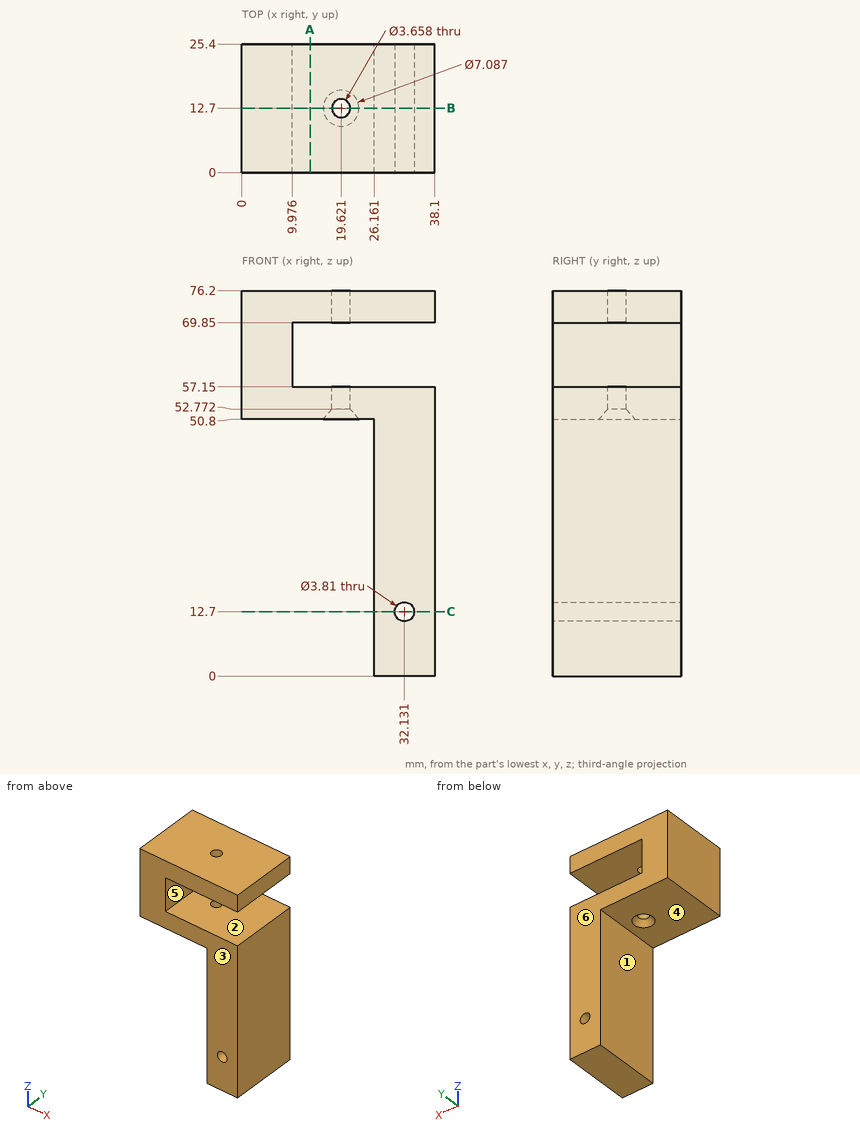
Part print with two shaded views. Sizes in mm from the minimum x, y, z corner. A direction names the side the tool comes from. Give positions to 0.01 mm unless a question says otherwise; leave off trailing zeros. Order: outer loops, then holes, each group sorted by start corner. A loop starts at its lowest first (then second) coordinate and runs counter-clockwise, first axis right, second up.
(1) Tool access for the marked faces 1, 2 and 3: list every direction of +Z, -Z, +X, -X, +Y, -Y with a clear straight run to the whole face (end or side of a thin tool).
(2) Saw through at C-C, the plane z = 12.7. Give the cut face in (x, y) (1 decimal).
(3) Saw through at A-A, the plane x = 13.5. Give the cut face in (y, z).
(4) Drill centre lines: L1, parallel to Z at x = 28, y = 15.25; L2, parallel to Z at x = 21.5, y = 16; L3, parallel to X at y = 6, z = 12.7 (1 decimal). Where is each one in solid material? Low to high.
(5) Flat gauge pins, fed straight in: pin 1 (10 mm diameter, centred on y = 13, z = 19, fed in from -X); pin 2 (12.5 mm diameter, centred on x = 11, y = 18.5, fed in from -Z); pin 3 (6.5 mm diameter, centred on y = 8, z = 65.5, fed in from +X). Where does each tip first touch, or does it go through?
(6) Mould opens along Z. For the marked faces 4, 5 and 6 say: released by +Z, released by -Z, zero draft, split by the parting line, or undercut.
(7) Saw through at B-B, the plane y = 12.7. State how many separate pieces and enclosed holes the cut face has, then the cut area to 3 significant figures.
Results found:
1. face 1: -Z, -X, +Y, -Y
1. face 2: +X, +Y, -Y
1. face 3: +Z, -Z, +X, -X, -Y
2. outline: (26.2, 0) - (30.2, 0) - (30.2, 25.4) - (26.2, 25.4) - close; (34, 0) - (38.1, 0) - (38.1, 25.4) - (34, 25.4) - close
3. outline: (0, 50.8) - (25.4, 50.8) - (25.4, 57.15) - (0, 57.15) - close; (0, 69.85) - (25.4, 69.85) - (25.4, 76.2) - (0, 76.2) - close
4. L1: z = 0 to 57.15, 69.85 to 76.2
4. L2: z = 50.8 to 57.15, 69.85 to 76.2
4. L3: x = 26.2 to 30.2, 34 to 38.1
5. pin 1: stops at x = 26.16
5. pin 2: stops at z = 50.8
5. pin 3: stops at x = 9.98
6. face 4: released by -Z
6. face 5: undercut
6. face 6: zero draft
7. separate pieces: 3
7. enclosed holes: 1
7. area: 1,160 mm2
